from build123d import *

# Parameters (mm, degrees)
SKETCH003_R  = 1.4
PAD003_DEPTH = 30
BOX013_W     = 54
BOX013_H     = 2
BOX013_DEPTH = 109
FILLET006_R  = 5


with BuildPart() as pad003:
    # Sketch003 → Pad003 (new body)
    with BuildSketch(Plane.XZ.offset(10)):
        with Locations((139, 116)):
            Circle(SKETCH003_R)
        with Locations((186, 116)):
            Circle(SKETCH003_R)
        with Locations((139, 14)):
            Circle(SKETCH003_R)
        with Locations((186, 14)):
            Circle(SKETCH003_R)
    extrude(amount=-PAD003_DEPTH)


with BuildPart() as cut008:
    # Box013 → Box013 (new body)
    with BuildSketch(Plane(origin=(135.5, 0, 10.5), x_dir=(1, 0, 0), z_dir=(0, 0, 1))):
        with Locations((27, 1)):
            Rectangle(BOX013_W, BOX013_H)
    extrude(amount=BOX013_DEPTH)

    # Fillet006
    fillet006_edges = [cut008.edges().sort_by_distance(p)[0] for p in [
        (135.5, 1, 119.5),
        (135.5, 1, 10.5),
        (189.5, 1, 119.5),
        (189.5, 1, 10.5),
    ]]
    fillet(fillet006_edges, radius=FILLET006_R)

    # Cut008: cut Pad003
    add(pad003.part, mode=Mode.SUBTRACT)


solid = cut008.part
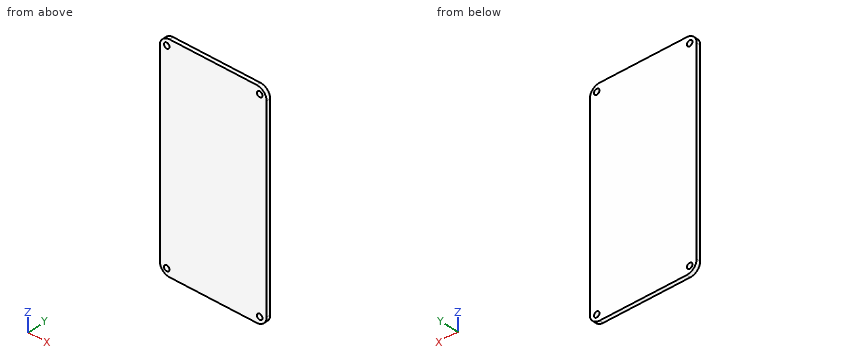
CAD build for the part. Positions are in the model's coordinates, mm. Round coordinates to 2 decimals unless told otherwise and drop trailing zeros. Loops run counter-clockwise (first coordinate to the right, second up) from the corner with the lowest first, then second, coordinate; pieces in that order, holes last.
(1) Cut at A-A (x = 139). Give the cut face in (y, z).
(2) Cut at B-B (z = 14). Give the cut face in (x, y).
(3) Wall check: line 1 along X through (y, z) = (1.6, 116); line 2 along Z through (x, y) = (185, 1.15); line 3 along Z through (x, y) = (186, 1.2). Give the ranges that are in metal, low to high.
Findings below:
1. outline: (0, 10.73) - (2, 10.73) - (2, 12.6) - (0, 12.6) - close; (0, 15.4) - (2, 15.4) - (2, 114.6) - (0, 114.6) - close; (0, 117.4) - (2, 117.4) - (2, 119.27) - (0, 119.27) - close
2. outline: (135.73, 0) - (137.6, 0) - (137.6, 2) - (135.73, 2) - close; (140.4, 0) - (184.6, 0) - (184.6, 2) - (140.4, 2) - close; (187.4, 0) - (189.27, 0) - (189.27, 2) - (187.4, 2) - close
3. line 1: x = 135.73 to 137.6, 140.4 to 184.6, 187.4 to 189.27
3. line 2: z = 10.53 to 13.02, 14.98 to 115.02, 116.98 to 119.47
3. line 3: z = 10.73 to 12.6, 15.4 to 114.6, 117.4 to 119.27
